Input: part model. Units: mm. Frame: model coordinates. A direction names the side the tool comes from. Round coordinates to 2 decimals unless told otherwise and drop trailing zeros. Loops run counter-clockwise (first coordinate to the right, second up) from the corner with the lowest first, then second, coordinate; pieces in that order, holes last. Notation, with made-up numbers: (89, 27) -> (138, 27) arc R19 ccw to (138, 42) -> close; hole circle Ø2 at (47, -29). An arc over 180 degrees is marked (long way). Answer as a JSON object with one key per item and string values. Group by question number.
Item 1: Section query B-B on z = -1.5. Return loops of the section in (x, y) (1 decimal), and give its area (3 significant figures).
Item 2: Set-up query: faces 1 (the flat face through (0, -2, 0)), 2 (the flat face through (21, 0, 0)), 3 (the flat face through (-21, 0, 0)), 4 (the flat face through (22.67, 0, -2)), 5 (the flat face through (0, 5.08, 1)). Return all of +Z, -Z, +X, -X, +Y, -Y with unobstructed straight access to the full face (end or side cutting, diameter ignored); none if empty.
Item 3: Pin query (flat end, axial travel): pin 1 (4 mm diameter, centred on x = 18.86, y = 0, fed in from +Z); pin 2 (4.5 mm diameter, centred on x = 0, y = 0, fed in from -Z); pin 3 (4 mm diameter, centred on y = 3.5, z = 2.5, fed in from -X); pin 4 (1.9 mm diameter, centred on x = -18.86, y = 0, fed in from -Z). Return the tip coordinate at first contact, or that it passes through.
Item 4: Material intervals for line 1 (X direction, y = -3, z = -0.25); line 2 (Z direction, x = 21, y = 3.25); line 3 (Z direction, x = -6, y = -2.5), sorted ascending. Write a range as [from, to].
Item 5: Section query A-A on x = 0. Return loops of the section in (y, z), and give its area (3 significant figures).
Item 6: Draft query along Y for faces 6 (the cylindrical face through (-1.525, -0.632, 1.878)), 7 (the cylindrical face through (20.41, 0.34, -1.93)), 8 (the flat face through (0, -2, 3.81)), 9 (the flat face through (0, -5.08, 1)). Return one class per face: released by +Y, released by -Y, zero draft, split by the parting line, or undercut.
Item 7: Section query D-D on z = 2.5. Return loops of the section in (x, y).
Item 8: Section query C-C on y = 0. Return loops of the section in (x, z), and give its area (3 significant figures).
Autodesk Inventor part; units mm, degrees
ref_plane "YZ Plane" through (0, 0, 0) normal (1, 0, 0) x (0, 1, 0)
ref_plane "XZ Plane" through (0, 0, 0) normal (0, 1, 0) x (-1, 0, 0)
ref_plane "XY Plane" through (0, 0, 0) normal (0, 0, 1) x (1, 0, 0)
sketch "Sketch1" plane through (0, 0, 0) normal (0, 0, 1) x (1, 0, 0)
  line L0 (-11.2395, -5.08) -> (11.2395, -5.08)
  line L1 (11.2395, -5.08) -> (11.2395, 5.08)
  line L2 (11.2395, 5.08) -> (-11.2395, 5.08)
  line L3 (-11.2395, 5.08) -> (-11.2395, -5.08)
  line L4 (-11.2395, -5.08) -> (11.2395, 5.08) construction
  line L5 (11.2395, -5.08) -> (-11.2395, 5.08) construction
  point P0 (0, 0)
  dimension "d0" = 22.479
  dimension "d1" = 10.16
extrude "Extrusion1" add sketch "Sketch1" along normal blind 3.81
sketch "Sketch2" plane through (0, 0, 3.81) normal (0, 0, 1) x (1, 0, 0)
  line L0 (11.2395, 5.08) -> (-11.2395, 5.08)
  line L1 (-11.2395, 5.08) -> (-15.0495, 5.08)
  line L2 (-15.0495, 5.08) -> (-15.0495, -5.08)
  line L3 (-15.0495, -5.08) -> (-11.2395, -5.08)
  line L4 (-11.2395, -5.08) -> (-11.2395, 5.08)
  line L5 (11.2395, -5.08) -> (11.2395, 5.08)
  line L6 (11.2395, 5.08) -> (15.0495, 5.08)
  line L7 (15.0495, 5.08) -> (15.0495, -5.08)
  line L8 (15.0495, -5.08) -> (11.2395, -5.08)
  line L9 (11.2395, -5.08) -> (11.2395, 5.08)
  point P0 (0, 0)
  dimension "d4" = 3.81
  dimension "d5" = 10.16
  dimension "d6" = 3.81
extrude "Extrusion2" add sketch "Sketch2" against normal blind 7.62
sketch "Sketch3" plane through (0, 0, -3.81) normal (0, 0, -1) x (-1, 0, 0)
  line L0 (-11.2395, -5.08) -> (-11.2395, 5.08)
  line L1 (-11.2395, 5.08) -> (-22.6695, 5.08)
  line L2 (-22.6695, 5.08) -> (-22.6695, -5.08)
  line L3 (-22.6695, -5.08) -> (-11.2395, -5.08)
  line L4 (-11.2395, -5.08) -> (-11.2395, 5.08)
  line L5 (11.2395, 5.08) -> (11.2395, -5.08)
  line L6 (11.2395, 5.08) -> (22.6695, 5.08)
  line L7 (22.6695, 5.08) -> (22.6695, -5.08)
  line L8 (22.6695, -5.08) -> (11.2395, -5.08)
  line L9 (11.2395, -5.08) -> (11.2395, 5.08)
  point P0 (0, 0)
  dimension "d9" = 11.43
  dimension "d10" = 10.16
  dimension "d11" = 11.43
  dimension "d12" = 10.16
extrude "Extrusion3" add sketch "Sketch3" against normal blind 3.81
sketch "Sketch4" plane through (0, 0, 0) normal (0, 0, -1) x (-1, 0, 0)
  circle A0 centre (0, 0) radius 1.651
  dimension "d15" = 3.302
extrude "Extrusion4" cut sketch "Sketch4" against normal through all
sketch "Sketch5" plane through (0, 0, 0) normal (0, 0, 1) x (1, 0, 0)
  line L0 (15.0495, -5.08) -> (22.6695, -5.08)
  line L1 (-22.6695, -5.08) -> (-15.0495, -5.08)
  line L2 (22.6695, -5.08) -> (22.6695, 5.08)
  line L3 (-22.6695, 5.08) -> (-22.6695, -5.08)
  point P0 (0, 0)
  point P1 (-18.8595, 0)
  point P2 (18.8595, 0)
  dimension "d18" = 5.08
  dimension "d19" = 5.08
  dimension "d20" = 3.81
  dimension "d21" = 3.81
hole "Hole1" at (-18.8595, 0, 0) at (18.8595, 0, 0) direction (0, 0, -1) diameter 3.175 end through all
fillet "Fillet1" radius 2.032 2 edges at (15.0495, 0, 0) (-15.0495, 0, 0)
properties part number "LowerSpringMount"
Solved:
{
 "1": {"outline": "(-22.7, -5.1) -> (-11.2, -5.1) -> (-11.2, 5.1) -> (-22.7, 5.1) -> close; (11.2, -5.1) -> (22.7, -5.1) -> (22.7, 5.1) -> (11.2, 5.1) -> close; hole circle Ø3.2 at (-18.9, 0); hole circle Ø3.2 at (18.9, 0)", "area": "216 mm²"},
 "2": {"face 1": "-Z, +Y, -Y", "face 2": "+Z, +X, +Y, -Y", "face 3": "+Z, -X, +Y, -Y", "face 4": "+Z, -Z, +X, +Y, -Y", "face 5": "+Z, -Z, +X, -X, +Y"},
 "3": {"pin 1": "z = 0.01", "pin 2": "z = 0", "pin 3": "x = -15.75", "pin 4": "through"},
 "4": {"line 1": "[-22.67, -11.24], [11.24, 22.67]", "line 2": "[-3.81, 0]", "line 3": "[0, 3.81]"},
 "5": {"outline": "(-5.08, 0) -> (-1.65, 0) -> (-1.65, 3.81) -> (-5.08, 3.81) -> close; (1.65, 0) -> (5.08, 0) -> (5.08, 3.81) -> (1.65, 3.81) -> close", "area": "26.1 mm²"},
 "6": {"face 6": "undercut", "face 7": "undercut", "face 8": "zero draft", "face 9": "released by -Y"},
 "7": {"outline": "(-15.05, -5.08) -> (15.05, -5.08) -> (15.05, 5.08) -> (-15.05, 5.08) -> close; hole circle Ø3.3 at (0, 0)"},
 "8": {"outline": "(-22.67, -3.81) -> (-20.45, -3.81) -> (-20.45, 0) -> (-22.67, 0) -> close; (-17.27, -3.81) -> (-11.24, -3.81) -> (-11.24, 0) -> (-1.65, 0) -> (-1.65, 3.81) -> (-15.05, 3.81) -> (-15.05, 2.03) arc R2.03 cw to (-17.08, 0) -> (-17.27, 0) -> close; (1.65, 0) -> (11.24, 0) -> (11.24, -3.81) -> (17.27, -3.81) -> (17.27, 0) -> (17.08, 0) arc R2.03 cw to (15.05, 2.03) -> (15.05, 3.81) -> (1.65, 3.81) -> close; (20.45, -3.81) -> (22.67, -3.81) -> (22.67, 0) -> (20.45, 0) -> close", "area": "167 mm²"}
}
